from build123d import *

# Parameters (mm, degrees)
SKETCH_1_R            = 1.55
SKETCH_1_R_2          = 1.05
SKETCH_1_R_3          = 1.581404189
SKETCH_1_W            = 8.2
SKETCH_1_H            = 15.5
SKETCH_1_H_2          = 16.001858204
EXTRUDE_1_DEPTH       = 1.6
SKETCH_1900_R         = 4.25
SKETCH_1900_R_2       = 2.5
CUT_EXTRUDE_5_DEPTH   = 85.317277267
EXTRUDE_3627_DEPTH    = 0.5
SKETCH_3_W            = 9.15
SKETCH_3_H            = 14.525
JST_GH_4PIN_X_2_DEPTH = 2.5
FILLET_3_R            = 2
EXTRUDE_START         = -1.6
EXTRUDE_5402_DEPTH    = 1.6


with BuildPart() as part:
    # 草图1 → 凸台-拉伸1 (new body)
    with BuildSketch(Plane(origin=(0, 0, 0), x_dir=(1, 0, 0), z_dir=(0, 1, 0))):
        Polygon((17.624917378, -7.723117708), (-4.691592189, -7.723117708), (-7.5, -10.531525519), (-7.5, -53.500834243), (-23.23198905, -53.500834243), (-23.23198905, -73.500834243), (22.7111878, -73.500834243), (22.7111878, -53.500834243), (7.5, -53.500834243), (7.5, -21.98577592), (12.62948765, -16.856288271), (17.315171978, -16.856288271), (20.682001416, -20.223117708), (26.774367048, -20.223117708), (29.820182402, -19.217148973), (29.820182402, 27.613551536), (22.124670003, 34.665102629), (18.4, 34.665102629), (6.35, 34.665102629), (7, 35.665102629), (7, 47.064038047), (6.331493599, 48.255532994), (29.1, 52.697797243), (30.35, 55.088888723), (30.35, 73.962756038), (29.042220737, 78.649353117), (20.842220737, 78.649353117), (19.65, 73.962756038), (19.65, 58.462756038), (-7, 52.009711353), (-7, 37.490925595), (0, 29.276882292), (17.314498575, 29.276882292), (19.254012403, 25.957144), (20.269436965, -6.007948815), align=None)
        with Locations(Location((0, -30.287243962, 0), (0, 0, 270))):
            Circle(SKETCH_1_R, mode=Mode.SUBTRACT)
        with Locations(Location((0, -50.787243962, 0), (0, 0, 270))):
            Circle(SKETCH_1_R, mode=Mode.SUBTRACT)
        with Locations(Location((25, 76.412756037, 0), (0, 0, 270))):
            Circle(SKETCH_1_R_2, mode=Mode.SUBTRACT)
        with Locations(Location((25, 56.012756039, 0), (0, 0, 270))):
            Circle(SKETCH_1_R_2, mode=Mode.SUBTRACT)
        with Locations(Location((23.5, -13.5, 0), (0, 0, 270))):
            Circle(SKETCH_1_R, mode=Mode.SUBTRACT)
        with Locations(Location((-16.865979253, -56.895287035, 0), (0, 0, 270))):
            Circle(SKETCH_1_R_3, mode=Mode.SUBTRACT)
        with Locations(Location((16.865979253, -56.895287035, 0), (0, 0, 270))):
            Circle(SKETCH_1_R, mode=Mode.SUBTRACT)
        with Locations((25, 66.212756038)):
            Rectangle(SKETCH_1_W, SKETCH_1_H, mode=Mode.SUBTRACT)
        with Locations((0, -40.536314862)):
            Rectangle(SKETCH_1_W, SKETCH_1_H_2, mode=Mode.SUBTRACT)
    extrude(amount=EXTRUDE_1_DEPTH)

    # Sketch 1900 → 切除-拉伸5 (cut, through all)
    with BuildSketch(Plane(origin=(0, 0, 0), x_dir=(1, 0, 0), z_dir=(0, 1, 0))):
        with BuildLine():
            ThreePointArc((32.25, -19.787243962), (31.591537652, -17.514941761), (29.820184804, -15.946745651))
            Line((29.820184804, -15.946745651), (29.820138471, -18.164164281))
            ThreePointArc((29.820138471, -18.164164281), (29.388960143, -16.929984913), (29.04688934, -15.668200055))
            ThreePointArc((29.04688934, -15.668200055), (24.645020142, -22.396192055), (32.25, -19.787243962))
        make_face()
        with BuildLine():
            Line((29.820138471, -18.164164281), (29.820184804, -15.946745651))
            ThreePointArc((29.820184804, -15.946745651), (29.440286586, -15.788734921), (29.04688934, -15.668200055))
            ThreePointArc((29.04688934, -15.668200055), (29.388960143, -16.929984913), (29.820138471, -18.164164281))
        make_face()
        with Locations((28, -19.787243962)):
            Circle(SKETCH_1900_R)
        with BuildLine():
            ThreePointArc((29.389676683, 28.446687445), (29.699958614, 29.863367854), (29.821172201, 31.308554874))
            Line((29.821172201, 31.308554874), (29.820138471, -18.164164281))
            ThreePointArc((29.820138471, -18.164164281), (28.692543787, -13.637691906), (28.744612063, -8.973175765))
            ThreePointArc((28.744612063, -8.973175765), (28.818369707, -6.611977276), (28.386269498, -4.289481227))
            ThreePointArc((28.386269498, -4.289481227), (27.36992989, -0.250862064), (26.720671038, 3.862756038))
            Line((26.720671038, 3.862756038), (26.610745663, 6.062756038))
            ThreePointArc((26.610745663, 6.062756038), (27.113818567, 17.364766035), (29.389676683, 28.446687445))
        make_face()
        with Locations((28, 36.212756038)):
            Circle(SKETCH_1900_R)
        with Locations((16.265283418, -5.723117708)):
            Circle(SKETCH_1900_R_2)
    extrude(amount=CUT_EXTRUDE_5_DEPTH, mode=Mode.SUBTRACT)

    # Sketch 2795 → Extrude 3627 (add)
    with BuildSketch(Plane(origin=(0, 0, 0), x_dir=(1, 0, 0), z_dir=(0, 1, 0))):
        Polygon((5.284716582, -7.723117708), (0.215283418, -7.723117708), (0.215283418, -19.223117708), (1.334716582, -19.223117708), (5.284716582, -15.273117708), align=None)
        Polygon((-0.215283418, -7.723117708), (-4.691592189, -7.723117708), (-5.284716582, -8.316242101), (-5.284716582, -19.223117708), (-0.215283418, -19.223117708), align=None)
    extrude(amount=-EXTRUDE_3627_DEPTH)

    # Sketch 3 → JST-GH-4Pin x 2 (add)
    with BuildSketch(Plane(origin=(0, 0, 0), x_dir=(1, 0, 0), z_dir=(0, 1, 0))):
        with Locations((15.075, 66.225256038)):
            Rectangle(SKETCH_3_W, SKETCH_3_H)
    extrude(amount=JST_GH_4PIN_X_2_DEPTH)

    # 圆角3
    # the kernel refuses this fillet: 2 mm, written as the material it adds along each edge
    with BuildSketch(Plane(origin=(19.65, 0, -58.962756038), x_dir=(0, 0, 1), z_dir=(0, 1, 0))) as fillet_3_piece_1:
        with BuildLine():
            CenterArc((2, -1.322875656), FILLET_3_R, 138.590377891, 41.409622109)
            Line((0, -1.322875656), (0, 0))
            Line((0, 0), (0.5, 0))
        make_face()
    extrude(amount=1.6)
    with BuildSketch(Plane(origin=(19.65, 0, -73.487756038), x_dir=(0, 0, -1), z_dir=(0, 1, 0))) as fillet_3_piece_2:
        with BuildLine():
            CenterArc((2, 1.293976429), FILLET_3_R, 180, 40.314909173)
            Line((0, 1.293976429), (0, 0))
            Line((0, 0), (0.475, 0))
        make_face()
    extrude(amount=1.6)
    with BuildSketch(Plane(origin=(7.5, 0, 53.500834243), x_dir=(0, 0, -1), z_dir=(0, 1, 0)), Plane(origin=(-7.5, 0, 53.500834243), x_dir=(-1, 0, 0), z_dir=(0, 1, 0))) as fillet_3_piece_3:
        with BuildLine():
            CenterArc((FILLET_3_R, -FILLET_3_R), FILLET_3_R, 90, 90)
            Line((0, -FILLET_3_R), (0, 0))
            Line((0, 0), (FILLET_3_R, 0))
        make_face()
    extrude(amount=1.6)
    # the kernel refuses this fillet: 2 mm, written as the material it takes off along each edge
    with BuildSketch(Plane(origin=(10.5, -5, -58.962756038), x_dir=(0, 0, -1), z_dir=(0, 1, 0)), Plane(origin=(10.5, -5, -73.487756038), x_dir=(1, 0, 0), z_dir=(0, 1, 0))) as fillet_3_2_piece_1:
        with BuildLine():
            CenterArc((FILLET_3_R, -FILLET_3_R), FILLET_3_R, 90, 90)
            Line((0, -FILLET_3_R), (0, 0))
            Line((0, 0), (FILLET_3_R, 0))
        make_face()
    extrude(amount=12.5, mode=Mode.SUBTRACT)
    with BuildSketch(Plane(origin=(-7, -3.933789701, -52.009711353), x_dir=(0.9719132109472551, 0, -0.23533956400528205), z_dir=(0, 1, 0))) as fillet_3_2_piece_2:
        with BuildLine():
            CenterArc((FILLET_3_R * 0.786757940299, -FILLET_3_R), FILLET_3_R, 90, 76.388360252)
            Line((-FILLET_3_R * 0.185155270648, -FILLET_3_R * 0.764660435995), (0, 0))
            Line((0, 0), (FILLET_3_R * 0.786757940299, 0))
        make_face()
    extrude(amount=9.467579403, mode=Mode.SUBTRACT)
    with BuildSketch(Plane(origin=(23.77241037, 6.158816797, 20.223117708), x_dir=(-1, 0, 0), z_dir=(0, -1, 0))) as fillet_3_2_piece_3:
        with BuildLine():
            CenterArc((1.823526719, 2), FILLET_3_R, 194.492910043, 75.507089957)
            ThreePointArc((-0.112830513, 1.499479599), (0.010429415, 0.754769623), (0, 0))
            Line((0, 0), (1.823526719, 0))
        make_face()
    extrude(amount=10.717633594, mode=Mode.SUBTRACT)
    with BuildSketch(Plane(origin=(-23.23198905, -5, 73.500834243), x_dir=(0, 0, -1), z_dir=(0, 1, 0)), Plane(origin=(22.7111878, -5, 73.500834243), x_dir=(-1, 0, 0), z_dir=(0, 1, 0)), Plane(origin=(22.7111878, -5, 53.500834243), x_dir=(0, 0, 1), z_dir=(0, 1, 0)), Plane(origin=(-23.23198905, -5, 53.500834243), x_dir=(1, 0, 0), z_dir=(0, 1, 0))) as fillet_3_2_piece_4:
        with BuildLine():
            CenterArc((FILLET_3_R, -FILLET_3_R), FILLET_3_R, 90, 90)
            Line((0, -FILLET_3_R), (0, 0))
            Line((0, 0), (FILLET_3_R, 0))
        make_face()
    extrude(amount=11.6, mode=Mode.SUBTRACT)
    with BuildSketch(Plane(origin=(29.290123585, 4.655582445, -28.099254974), x_dir=(-0.26492584299558386, 0, 0.9642687891418446), z_dir=(0, -1, 0))) as fillet_3_2_piece_5:
        with BuildLine():
            CenterArc((1.222348791, 1.99992922), FILLET_3_R, 207.137102211, 62.380861619)
            Line((-0.557486463, 1.087686672), (0, 0))
            ThreePointArc((0, 0), (0.602761377, 0.002535566), (1.205522753, 0))
        make_face()
    extrude(amount=7.71116489, mode=Mode.SUBTRACT)
    with BuildSketch(Plane(origin=(29.04688934, 7.189707678, 15.668200055), x_dir=(-0.9998305759549154, 0, -0.018407047173896997), z_dir=(0, -1, 0))) as fillet_3_2_piece_6:
        with BuildLine():
            CenterArc((2.398675677, 1.947113498), FILLET_3_R, 172.818157219, 83.976285302)
            ThreePointArc((0.414366937, 2.197151144), (0.240731561, 1.092248642), (0, 0))
            ThreePointArc((0, 0), (0.970892536, 0.112383816), (1.941785072, 0))
        make_face()
    extrude(amount=12.779415356, mode=Mode.SUBTRACT)

    # Sketch 3 2 → Extrude 5402 (add)
    with BuildSketch(Plane(origin=(0, 1.6, 0), x_dir=(1, 0, 0), z_dir=(0, 1, 0)).offset(EXTRUDE_START)):
        Polygon((-13.766428784, 32.326134419), (-10.943503558, 29.013615841), (-0.308926004, 29.013615841), (0, 29.276882292), (-7, 37.490925595), (-7, 38.092478683), align=None)
    extrude(amount=EXTRUDE_5402_DEPTH)


solid = part.part
Verification items for the finished model (mm, model axes). A direction names the side the tool comes from. Coordinates: 2 decimals unless noted, no trailing zeros. Write each loop counter-clockwise with the first axis right and the second up, starting at its lowest first coordinate (ties: lowest second). Pieces come first, ordered by that corner, then holes. Notation, with made-up numbers: (-8, -24) -> (38, -24) arc R24 cw to (38, 11) -> close; hole circle Ø8 at (-32, 84.25). An arc over 180 degrees is marked (long way). One line per item, written item: value. Start each with the question number.
Q1. Thickness scan on L1, parallel to X at y = 0.8, z = 46; L2, parallel to Z at x = 9, y = 1.2; L3, parallel to Y at x = 25.5, z = -12. Record the ranges inside material, lowest first. Write a range as from..to.
Q2. Go/stop test with flat-tipped pins: P1, Ø0.6, axis at x = 0.5, y = -0.5, coming from the +Z side; P2, Ø0.6, axis at y = 0, z = 12, coming from the +X side; P3, Ø0.8, axis at y = 1, z = -65, coming from the -X side. Record where each tip stops, or that it passes through.
Q3. Cross-section at A-A on z = -41. Enter the section's corners in (x, y), and give its area (3 significant figures).
Q4. Access from +Z, -Z, +X, -X, +Y, -Y to the whole of each face (thin tool, end or side, straight path). Record for faces 1 (the flat face through (7.266, 0.789, -55.464)), 2 (the flat face through (10.5, 1, -66)), 3 (the flat face through (25.301, 0.789, -31.755)), 4 (the flat face through (18.98, 0.79, 18.52)).
Q5. Mould release check, pull along X, two halves, no side actions. Record for faces 5 (the flat face through (15, 1, -58.963)), 6 (the flat face through (10.029, 0.789, 19.457)), 7 (the flat face through (3.28, -0.25, 17.28)): pulls with the +X half, pulls with the -X half, needs draft (parallel to the pull), parting line crosses it, or undercut.
Checked values:
1. L1: x = -7.5..-4.1, 4.1..7.5
1. L2: z = -55.88..-48.78, -34.67..-29.28, 7.72..20.49, 53.44..73.5
1. L3: y = 0..1.6
2. P1: stops at z = 19.22
2. P2: stops at x = 28.59
2. P3: stops at x = 10.5
3. outline: (-7, 0) -> (7, 0) -> (7, 1.6) -> (-7, 1.6) -> close
3. area: 22.4 mm²
4. face 1: -X, +Y, -Y
4. face 2: -Z, -X, +Y, -Y
4. face 3: +X, +Y, -Y
4. face 4: +Y, -Y
5. face 5: needs draft
5. face 6: undercut
5. face 7: pulls with the +X half
